Verification items for this drawing (mm, ordinates from the low corner). A direction names the side the tool comes from. Round coordinates to 2 decimals unless told otherwise and drop trailing zeros. Order: outer loops, then holes, each group sorted by start corner. A loop starts at its lowest first (then second) coordinate and runs counter-clockwise, first axis right, second up. Notation, with made-up numbers: (80, 87.25) - (129, 87.25) arc R16 ccw to (129, 97.25) - close; hole circle Ø8 at (17.25, -26.75). An arc over 180 degrees is marked (long way). Use a Markdown table: item, result. Add a question column.
(1) Section check B-B on x = 209. Record the boundary of the cut face in (y, z).
(2) Thickness scan on line 1 along X through (y, z) = (166, 14.5); line 2 along Y through (x, z) = (139.5, 9); line 3 along Y through (x, z) = (126, 10). Record the ranges inside material, lowest first. Write a range as [from, to].
(3) Gauge pin test, flat ends, axial feed: P1, Ø15, axis at x = 73.5, z = 13, coming from the +Y side; P2, Ø8, axis at y = 50, z = 17.5, coming from the -X side; P3, Ø6, axis at y = 29, z = 7, coming from the +X side. Record the tip position at first contact, or that the pin passes through.
(4) Access from +Z, -Z, +X, -X, +Y, -Y to the whole of each face (thin tool, end or side, straight path). Record for the marked faces 1 and 2.
(5) Section check A-A on y = 150. Record the boundary of the cut face in (x, z), then the cut area to 3 significant figures.
(6) Section check D-D on x = 180.5. Record the boundary of the cut face in (y, z), then the cut area to 3 significant figures.
(7) Section check C-C on y = 114. Record the boundary of the cut face in (x, z).
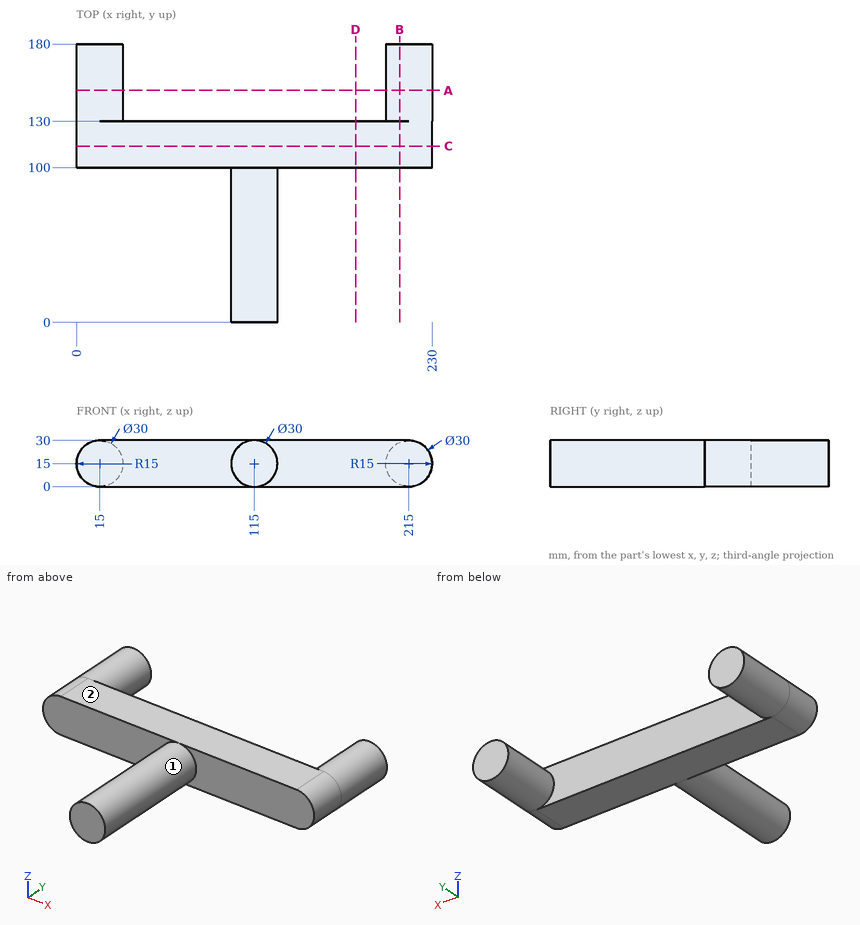
Check sheet entries:
| question | item | result |
|---|---|---|
| 1 | outline | (100, 0) - (130, 0) - (130, 1.25) - (180, 1.25) - (180, 28.75) - (130, 28.75) - (130, 30) - (100, 30) - close |
| 2 | line 1 | x = [0.01, 29.99], [200.01, 229.99] |
| 2 | line 2 | y = [100, 130] |
| 2 | line 3 | y = [0, 130] |
| 3 | P1 | stops at y = 130 |
| 3 | P2 | stops at x = 100 |
| 3 | P3 | stops at x = 129.14 |
| 4 | face 1 | -Y |
| 4 | face 2 | +Z, +X, -X, +Y, -Y |
| 5 | outline | circle Ø30 at (15, 15); circle Ø30 at (215, 15) |
| 5 | area | 1,410 mm2 |
| 6 | outline | (100, 0) - (130, 0) - (130, 30) - (100, 30) - close |
| 6 | area | 900 mm2 |
| 7 | outline | (15, 0) - (215, 0) arc R15 ccw to (215, 30) - (15, 30) arc R15 ccw to start |
